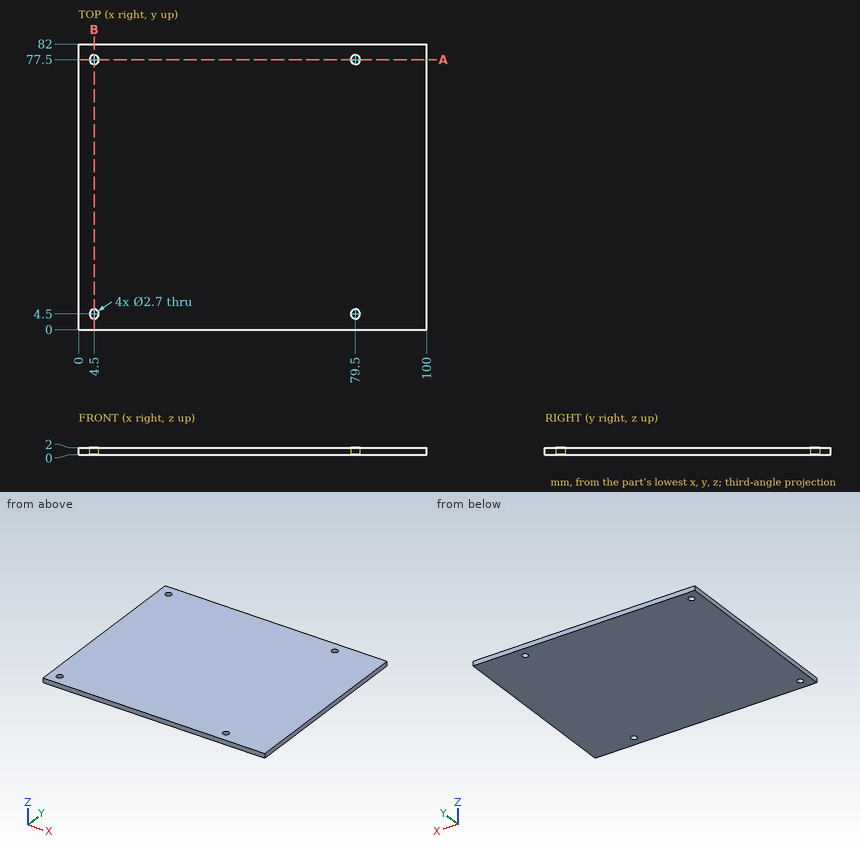
Source: three-view drawing plus pictorial views. Frame: mm from the lowest corner of the part. Coordinates: 2 decimals unless noted, no trailing zeros. Loops run counter-clockwise (first coordinate to the right, second up) from the corner with the lowest first, then second, coordinate; pieces in that order, holes last. Notation, with made-up numbers: (27, 32) -> (38, 32) arc R24 cw to (38, 60) -> close; hole circle Ø11 at (36, 61). An arc over 180 degrees is marked (long way). Answer in a Markdown table with one row per item. Add a question column.
Q1. Section B-B on x = 4.5. Return the cut outline in (y, z).
Q2. Ray query, line 1 along X through (y, z) = (4.5, 1.1); line 2 along Y through (x, z) = (79.5, 1.6); line 3 along Y through (x, z) = (5.5, 0.8). Return the intervals inside material, ascending.
Q3. Section A-A on y = 77.5. Return the cut outline in (x, z).
Q4. Contact query for a flat-ended pin moving along its axis: pin 1 Ø3.5 at (x, y) = (79.5, 77.5) entering from -Z. Output: stop coordinate, or through.
Computed values:
| question | item | result |
|---|---|---|
| 1 | outline | (0, 0) -> (3.15, 0) -> (3.15, 2) -> (0, 2) -> close; (5.85, 0) -> (76.15, 0) -> (76.15, 2) -> (5.85, 2) -> close; (78.85, 0) -> (82, 0) -> (82, 2) -> (78.85, 2) -> close |
| 2 | line 1 | x = 0 to 3.15, 5.85 to 78.15, 80.85 to 100 |
| 2 | line 2 | y = 0 to 3.15, 5.85 to 76.15, 78.85 to 82 |
| 2 | line 3 | y = 0 to 3.59, 5.41 to 76.59, 78.41 to 82 |
| 3 | outline | (0, 0) -> (3.15, 0) -> (3.15, 2) -> (0, 2) -> close; (5.85, 0) -> (78.15, 0) -> (78.15, 2) -> (5.85, 2) -> close; (80.85, 0) -> (100, 0) -> (100, 2) -> (80.85, 2) -> close |
| 4 | pin 1 | stops at z = 0 |
